Here's the drawing with two shaded views (mm, measured from the low corner). I have some questions. A direction names the side the tool comes from. Give positions to 0.01 mm unless a question says otherwise; leave off trailing zeros. Write each loop counter-clockwise with the first axis right and the second up, starting at its lowest first coordinate (ties: lowest second). Pieces come first, ordered by that corner, then holes.
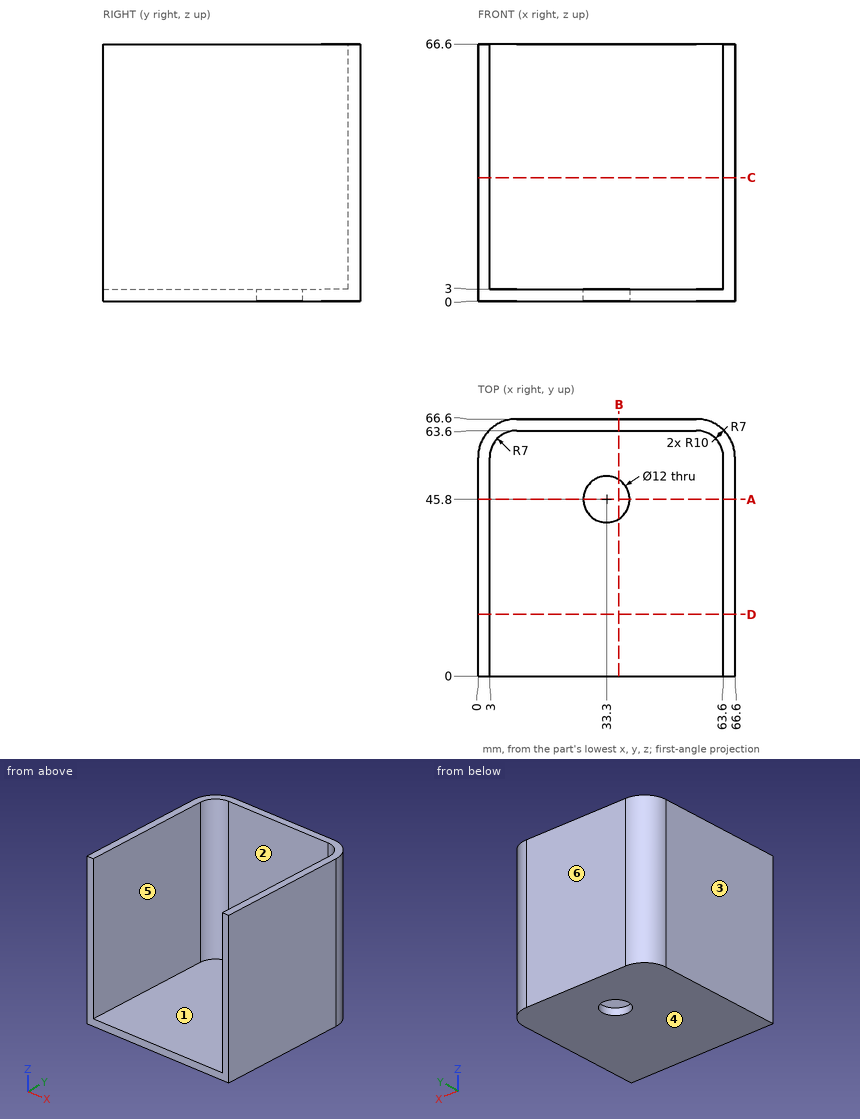
(1) If I drill on L1, parallel to X at y = 22, z = 22; L2, parallel to Y at x = 33.3, z = 1.8; L3, parallel to Z at x = 42.5, y = 54.5, over which ranges is the centre line in solid material (lowest first)?
Returned:
L1: x = 0 to 3, 63.6 to 66.6
L2: y = 0 to 39.8, 51.8 to 66.6
L3: z = 0 to 3
(2) Imagine slicing it at B-B, the plane x = 36.5. Write out the boundary of the cut face in (y, z).
Returned:
outline: (0, 0) - (40.72, 0) - (40.72, 3) - (0, 3) - close; (50.88, 0) - (66.6, 0) - (66.6, 66.6) - (63.6, 66.6) - (63.6, 3) - (50.88, 3) - close
(3) Will these pins go through, and if not, where does the flat tip stop? P1, Ø1, axis at x = 8.5, y = 31, coming from the +Z side; P2, Ø2, axis at x = 58, z = 46, coming from the +Y side; P3, Ø1.5, axis at x = 20.5, z = 34, coming from the -Y side.
Returned:
P1: stops at z = 3
P2: stops at y = 66.59
P3: stops at y = 63.6
(4) Imagine slicing it at A-A, the plane y = 45.8. Write out the boundary of the cut face in (x, z).
Returned:
outline: (0, 0) - (27.3, 0) - (27.3, 3) - (3, 3) - (3, 66.6) - (0, 66.6) - close; (39.3, 0) - (66.6, 0) - (66.6, 66.6) - (63.6, 66.6) - (63.6, 3) - (39.3, 3) - close
(5) If we mould it in two halves opening along X, with no side actions, what happens to the marked faces 1, 2, 3 and 4? For each: +X half, -X half, draft (parallel to the pull), parting line (faces both ways), or undercut.
Returned:
face 1: undercut
face 2: undercut
face 3: -X half
face 4: draft
(6) Imagine slicing it at D-D, the plane y = 16. Write out the boundary of the cut face in (x, z), plus the area to 3 significant figures.
Returned:
outline: (0, 0) - (66.6, 0) - (66.6, 66.6) - (63.6, 66.6) - (63.6, 3) - (3, 3) - (3, 66.6) - (0, 66.6) - close
area: 581 mm2
(7) Imagine slicing it at C-C, the plane z = 32. Write out the boundary of the cut face in (x, y).
Returned:
outline: (0, 0) - (3, 0) - (3, 56.6) arc R7 cw to (10, 63.6) - (56.6, 63.6) arc R7 cw to (63.6, 56.6) - (63.6, 0) - (66.6, 0) - (66.6, 56.6) arc R10 ccw to (56.6, 66.6) - (10, 66.6) arc R10 ccw to (0, 56.6) - close
(8) For the marked faces 5 and 6, which set-ups out of +Z, -Z, +X, -X, +Y, -Y let a thin tool reach every point of the face, with its end or its side?
Returned:
face 5: +Z, -Y
face 6: +Z, -Z, +X, -X, +Y
